Geometry check sheet. Reference: the model listing, model coordinates, mm. A direction names the side the tool comes from. Coordinates: 2 decimals unless noted, no trailing zeros. Loops run counter-clockwise (first coordinate to the right, second up) from the corner with the lowest first, then second, coordinate; pieces in that order, holes last. Notation, with made-up numbers: (36, 78) - (84, 78) arc R5 ccw to (84, 82) - close; hole circle Ø5 at (37, -22.5). An arc over 180 degrees is marked (long way). One line per item, written item: value.
from build123d import *

# Parameters (mm, degrees)
SKETCH_1_R             = 4.5
SKETCH_1_R_2           = 4
EXTRUDE_1_DEPTH        = 1.5
EXTRUDE_1_DEPTH_BACK   = 1.5
SKETCH_1_R_3           = 3
SKETCH_1_R_4           = 2.5
EXTRUDE_1_2_DEPTH      = 1.5
EXTRUDE_1_2_DEPTH_BACK = 1.5
SKETCH_2_R             = 4
SKETCH_2_R_2           = 3
EXTRUDE_2_DEPTH        = 1.2
EXTRUDE_2_DEPTH_BACK   = 1.2


with BuildPart() as part:
    # Sketch 1 → Extrude 1 (new body, two sides)
    with BuildSketch(Plane(origin=(0, 0, 0), x_dir=(1, 0, 0), z_dir=(0, 1, 0))) as extrude_1_sk:
        Circle(SKETCH_1_R)
        Circle(SKETCH_1_R_2, mode=Mode.SUBTRACT)
    extrude(amount=EXTRUDE_1_DEPTH)
    extrude(extrude_1_sk.sketch, amount=-EXTRUDE_1_DEPTH_BACK)



with BuildPart() as body_2:
    # Sketch 1 → Extrude 1 2 (new body, two sides)
    with BuildSketch(Plane(origin=(0, 0, 0), x_dir=(1, 0, 0), z_dir=(0, 1, 0))) as extrude_1_2_sk:
        Circle(SKETCH_1_R_3)
        Circle(SKETCH_1_R_4, mode=Mode.SUBTRACT)
    extrude(amount=EXTRUDE_1_2_DEPTH)
    extrude(extrude_1_2_sk.sketch, amount=-EXTRUDE_1_2_DEPTH_BACK)


with BuildPart() as part_1:
    add(part.part)

    add(body_2.part)  # Extrude 2 merges body 2
    # Sketch 2 → Extrude 2 (add, two sides)
    with BuildSketch(Plane(origin=(0, 0, 0), x_dir=(1, 0, 0), z_dir=(0, 1, 0))) as extrude_2_sk:
        Circle(SKETCH_2_R)
        Circle(SKETCH_2_R_2, mode=Mode.SUBTRACT)
    extrude(amount=EXTRUDE_2_DEPTH)
    extrude(extrude_2_sk.sketch, amount=-EXTRUDE_2_DEPTH_BACK)


solid = part_1.part
(1) Cross-section at D-D on x = 3.75. Record the cut outline in (y, z), and give its area (3 significant figures).
Reply:
outline: (-1.5, -2.49) - (1.5, -2.49) - (1.5, -1.39) - (1.2, -1.39) - (1.2, 1.39) - (1.5, 1.39) - (1.5, 2.49) - (-1.5, 2.49) - (-1.5, 1.39) - (-1.2, 1.39) - (-1.2, -1.39) - (-1.5, -1.39) - close
area: 13.3 mm2
(2) Cross-section at A-A on x = 0. Record the cut outline in (y, z).
Reply:
outline: (-1.5, -4.5) - (1.5, -4.5) - (1.5, -4) - (1.2, -4) - (1.2, -3) - (1.5, -3) - (1.5, -2.5) - (-1.5, -2.5) - (-1.5, -3) - (-1.2, -3) - (-1.2, -4) - (-1.5, -4) - close; (-1.5, 2.5) - (1.5, 2.5) - (1.5, 3) - (1.2, 3) - (1.2, 4) - (1.5, 4) - (1.5, 4.5) - (-1.5, 4.5) - (-1.5, 4) - (-1.2, 4) - (-1.2, 3) - (-1.5, 3) - close
(3) Cross-section at B-B on z = -1. Record the cut outline in (x, y), and give its area (3 significant figures).
Reply:
outline: (-4.39, -1.5) - (-3.87, -1.5) - (-3.87, -1.2) - (-2.83, -1.2) - (-2.83, -1.5) - (-2.29, -1.5) - (-2.29, 1.5) - (-2.83, 1.5) - (-2.83, 1.2) - (-3.87, 1.2) - (-3.87, 1.5) - (-4.39, 1.5) - close; (2.29, -1.5) - (2.83, -1.5) - (2.83, -1.2) - (3.87, -1.2) - (3.87, -1.5) - (4.39, -1.5) - (4.39, 1.5) - (3.87, 1.5) - (3.87, 1.2) - (2.83, 1.2) - (2.83, 1.5) - (2.29, 1.5) - close
area: 11.3 mm2
(4) Material ranges on probe 1 along X at (y, z) = (1.45, 0); probe 2 along Z at (x, y) = (0, -0.1), recorded low to high. Write a range as from..to.
Reply:
probe 1: -4.5..-4, -3..-2.5, 2.5..3, 4..4.5
probe 2: -4.5..-2.5, 2.5..4.5
(5) Cross-section at C-C on y = 0.9. Record the cut outline in (x, z), and give its area (3 significant figures).
Reply:
outline: circle Ø9 at (0, 0); hole circle Ø5 at (0, 0)
area: 44.0 mm2
(6) Access from +Z, -Z, +X, -X, +Y, -Y to the whole of each face (thin tool, end or side, straight path). Record for faces 1 (the face through (-0.54, -0.02, 2.44)), 2 (the face through (1, 1.2, -3)), 3 (the face through (1, -1.2, -3)).
Reply:
face 1: +Y, -Y
face 2: +Y
face 3: -Y
(7) Go/stop test with a flat-tipped pin: pin 1 Ø1.5 at (x, y) = (-3.5, 0) entering from +Z. Record where the tip stops, or that it passes through.
Reply:
pin 1: z = 3.56
(8) Release check for a two-part mould opening along Z. For faces 4 (the face through (-0.59, 0.02, -4.46)), 5 (the face through (-2, -1.5, -2)), 6 (the face through (-0.65, -1.35, 2.93)) record: pulls with the +Z half, pulls with the -Z half, needs draft (parallel to the pull), parting line crosses it, or undercut.
Reply:
face 4: parting line crosses it
face 5: needs draft
face 6: undercut
